Can you work these out from the drawing? Everything is in mm from the part's minimum corner. Give positions to 0.01 mm unless a question says otherwise; leave off trailing zeros. Loops run counter-clockwise (first coordinate to the right, second up) from the corner with the lowest first, then second, coordinate; pieces in that order, holes last.
Q1. If we section it at B-B (x = 58.5): Please give me the cut outline in (y, z).
Q2. If we section it at C-C (x = 44.5): Please give me the cut outline in (y, z), plus the area to 3 significant figures.
Q3. If we section it at A-A (y = 27): Please give me the cut outline in (x, z) (1 decimal).
Q4. Will these pins go through, and if not, where does the flat tip stop? P1, Ø8, axis at x = 29.5, y = 10.5, coming from the +Z side; P2, Ø10, axis at x = 61, y = 17, coming from the +Z side.
Q5. I need wall thicknesses on line 1 (X direction, y = 16.5, z = 133.5) (1 decimal); line 2 (X direction, y = 6, z = 139) (1 decimal); line 3 (Z direction, x = 74, y = 22.5). Which ranges of each line are inside material? Lowest first, please.
Q6. We'd pull the mould along X, two halves only. Please class the marked faces 1, 2, 3 and 4: +X half, -X half, draft (parallel to the pull), parting line (faces both ways), or undercut.
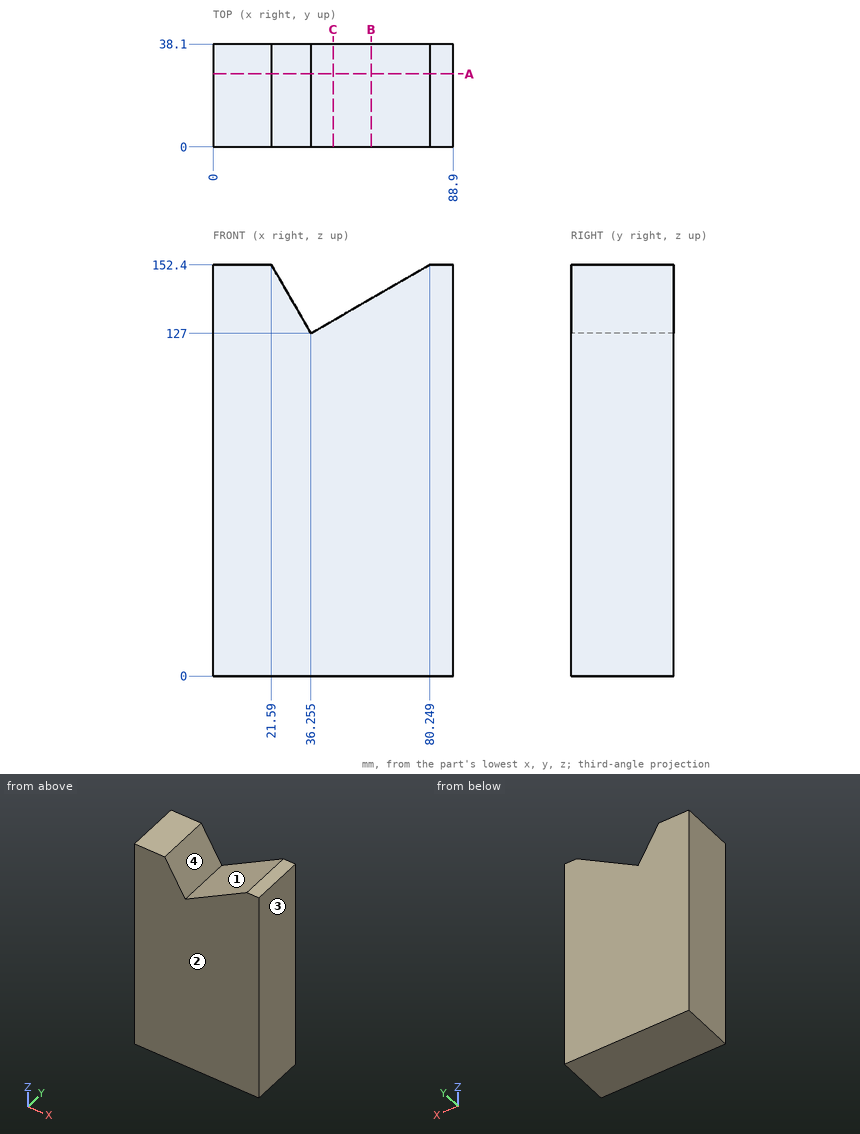
Check sheet entries:
1. outline: (0, 0) - (38.1, 0) - (38.1, 139.84) - (0, 139.84) - close
2. outline: (0, 0) - (38.1, 0) - (38.1, 131.76) - (0, 131.76) - close
2. area: 5,020 mm2
3. outline: (0, 0) - (88.9, 0) - (88.9, 152.4) - (80.2, 152.4) - (36.3, 127) - (21.6, 152.4) - (0, 152.4) - close
4. P1: stops at z = 145.63
4. P2: stops at z = 144.17
5. line 1: x = 0 to 32.5, 47.5 to 88.9
5. line 2: x = 0 to 29.3, 57 to 88.9
5. line 3: z = 0 to 148.79
6. face 1: undercut
6. face 2: draft
6. face 3: +X half
6. face 4: undercut
